Autodesk Inventor part; units mm, degrees
ref_plane "Start Plane" through (0, 0, 25) normal (0, 0, 1) x (1, 0, 0)
ref_plane "End Plane" through (0, 0, 450) normal (0, 0, 1) x (1, 0, 0)
ref_plane "Work Plane4" through (21, -20, 25) normal (0, 0, -1) x (-1, 0, 0)
ref_plane "Start Plane" through (0, 0, 25) normal (0, 0, 1) x (1, 0, 0)
ref_plane "End Plane" through (0, 0, 450) normal (0, 0, 1) x (1, 0, 0)
sketch "Sketch" plane through (0, 0, 0) normal (0, 0, 1) x (1, 0, 0)
  line L0 (-25, -41) -> (-25, 41)
  line L1 (-21, 45) -> (21, 45)
  line L2 (25, 41) -> (25, -41)
  line L3 (21, -45) -> (-21, -45)
  arc A0 (-25, -41) -> (-21, -45) centre (-21, -41) ccw
  arc A1 (25, 41) -> (21, 45) centre (21, 41) ccw
  arc A2 (-21, 45) -> (-25, 41) centre (-21, 41) ccw
  arc A3 (21, -45) -> (25, -41) centre (21, -41) ccw
  arc A4 (-21, 43) -> (-23, 41) centre (-21, 41) ccw
  line L4 (-21, 43) -> (21, 43)
  arc A5 (23, 41) -> (21, 43) centre (21, 41) ccw
  line L5 (23, 41) -> (23, -41)
  arc A6 (21, -43) -> (23, -41) centre (21, -41) ccw
  line L6 (21, -43) -> (-21, -43)
  arc A7 (-23, -41) -> (-21, -43) centre (-21, -41) ccw
  line L7 (-23, -41) -> (-23, 41)
  line L8 (0, 64.1598) -> (0, -64.1598) construction
  line L9 (-36.1598, 0) -> (36.1598, 0) construction
  dimension "d7" = 4
  dimension "d9" = 50
  dimension "d11" = 90
  dimension "d12" = 2
  dimension "d15" = 25
  dimension "d16" = 45
extrude "Body" add sketch "Sketch" along normal up to surface (425 mm away) from surface at 25
sketch "Sketch3" plane through (0, 0, 0) normal (0, 0, 1) x (1, 0, 0)
  line L0 (0, 0) -> (10, 0)
ref_plane "Work Plane3" through (0, 0, 0) normal (0, -1, 0) x (1, 0, 0)
sketch "Sketch4" plane through (0, 0, 0) normal (0, -1, 0) x (1, 0, 0)
  line L0 (-2, 25) -> (12, 25)
  line L1 (-2, 450) -> (12, 450)
  dimension "d18" = 425
ref_plane "Work Plane4" through (21, -20, 25) normal (0, 0, -1) x (-1, 0, 0)
split "Split1" plane through (21, -20, 25) removes the side toward (0, 0, -1)
sketch "Sketch5" plane through (25, -41, 450) normal (1, 0, 0) x (0, 0, -1)
  line L0 (425, 82) -> (425, 0)
  line L1 (295, 61) -> (355, 61)
  line L2 (355, 61) -> (355, 21)
  line L3 (355, 21) -> (295, 21)
  line L4 (295, 21) -> (295, 61)
  line L5 (425, 41) -> (406.5114, 41)
  point P0 (450, 41)
  dimension "d19" = 60
  dimension "d20" = 40
  dimension "d21" = 70
hole "Hole1" at (25, 20, 155) at (25, -20, 155) at (25, -20, 95) at (25, 20, 95) direction (-1, 0, 0) diameter 6.8 end through all
equation "\"d7\" = G_IR"
equation "\"d9\" = G_W"
equation "\"d11\" = G_H"
equation "\"d12\" = G_T"
equation "\"d15\" = 0.5 * d9"
equation "\"d16\" = 0.5 * d11"
equation "\"d3\" = G_L"
equation "\"G_W\" = 50"
equation "\"G_H\" = 90"
equation "\"G_T\" = 2"
equation "\"G_IR\" = 4"
equation "\"G_L\" = d18"
equation "\"G_OFFSET_START\" = -25"
equation "\"G_OFFSET_END\" = 0"
equation "\"d13\" = -G_OFFSET_START"
properties part number "ISO 10799-2 - 90x50x2 - 425" material "Steel, Mild"
The listing builds one solid part. Answer for the finished solid, in the listing's coordinates (mm). A direction names the side the tool comes from. Round coordinates to 2 decimals unless told otherwise and drop trailing zeros. Order: outer loops, then holes, each group sorted by start corner. A loop starts at its lowest first (then second) coordinate and runs counter-clockwise, first axis right, second up. Notation, with made-up numbers: M 3.5,29 L 34.5,29 A6 ccw 34.5,36 Z; hole C -33,76.25 d10. An arc over 180 degrees is marked long. Answer in a Markdown table with one row per item. Add a question column.
1) Consider line 1 along Z through (x, y) = (-23.85, -20); line 2 along Y through (x, z) = (-17.5, 87); line 3 along Y through (x, z) = (-21.5, 324). Determine where each line is inside the solid, lowest interval first. Write a range as from..to.
2) Which of the six approach directions +Z, -Z, +X, -X, +Y, -Y give full straight-line access (tool end or side, diameter ignored) to faces 1 (the face through (-24, 19.9, 158.4)), 2 (the face through (23, 1, 235))?
3) The part is cut by section B-B on z = 411. Determine the outline of the cut face in (x, y).
4) The part is cut by section A-A on y = -36.5. Determine the outline of the cut face in (x, z), plus the area to 3 significant figures.
5) The part is cut by section C-C on x = 12. Determine the outline of the cut face in (y, z).
6) Determine the mould class of faces 3 (the face through (0, 45, 235)), 4 (the face through (23.986, 22.069, 97.698)), 5 (the face through (-24, 0, 25)) for opening direction Y: pulls with the +Y half, pulls with the -Y half, needs draft (parallel to the pull), parting line crosses it, or undercut.
Findings below:
| question | item | result |
|---|---|---|
| 1 | line 1 | z = 25..91.6, 98.4..151.6, 158.4..450 |
| 1 | line 2 | y = -45..-43, 43..45 |
| 1 | line 3 | y = -44.97..-42.94, 42.94..44.97 |
| 2 | face 1 | +X, -X |
| 2 | face 2 | +Z, -Z |
| 3 | outline | M -25,-41 A4 ccw -21,-45 L 21,-45 A4 ccw 25,-41 L 25,41 A4 ccw 21,45 L -21,45 A4 ccw -25,41 Z; hole M -23,-41 A2 ccw -21,-43 L 21,-43 A2 ccw 23,-41 L 23,41 A2 ccw 21,43 L -21,43 A2 ccw -23,41 Z |
| 4 | outline | M -25,25 L -23,25 L -23,450 L -25,450 Z; M 23,25 L 25,25 L 25,450 L 23,450 Z |
| 4 | area | 1,700 mm² |
| 5 | outline | M -45,25 L -43,25 L -43,450 L -45,450 Z; M 43,25 L 45,25 L 45,450 L 43,450 Z |
| 6 | face 3 | pulls with the +Y half |
| 6 | face 4 | undercut |
| 6 | face 5 | needs draft |
